```python
from build123d import *

# Parameters (mm, degrees)
SKETCH1_R                 = 26
SKETCH1_R_2               = 17
BOSS_EXTRUDE1_DEPTH       = 6
FILLET1_R                 = 0.2
CUT_EXTRUDE1_START        = 18
SKETCH4_R                 = 2
CUT_EXTRUDE1_DEPTH        = 12
CIRPATTERN1_COUNT         = 6
LPATTERN1_COUNT           = 2
LPATTERN1_PITCH           = 6
LPATTERN1_START           = 18
LPATTERN1_COPY_1_SKETCH_R = 2
LPATTERN1_COPY_1_DEPTH    = 12
LPATTERN1_COPY_2_SKETCH_R = 2
LPATTERN1_COPY_2_DEPTH    = 12
LPATTERN1_COPY_3_SKETCH_R = 2
LPATTERN1_COPY_3_DEPTH    = 12
LPATTERN1_COPY_4_SKETCH_R = 2
LPATTERN1_COPY_4_DEPTH    = 12
LPATTERN1_COPY_5_SKETCH_R = 2
LPATTERN1_COPY_5_DEPTH    = 12


with BuildPart() as part:
    # Sketch1 → Boss-Extrude1 (new, symmetric)
    with BuildSketch(Plane(origin=(0, 0, 0), x_dir=(1, 0, 0), z_dir=(0, 1, 0))):
        with Locations(Location((0, 0, 0), (0, 0, 270))):
            Circle(SKETCH1_R)
        with Locations(Location((0, 0, 0), (0, 0, 270))):
            Circle(SKETCH1_R_2, mode=Mode.SUBTRACT)
    extrude(amount=BOSS_EXTRUDE1_DEPTH, both=True)

    # Sketch3 → Cut-Revolve1 (revolve, cut)
    with BuildSketch(Plane.XY, mode=Mode.PRIVATE) as cut_revolve1_sk:
        Polygon((-26, 0.2), (-26, -0.2), (-25.8, 0), align=None)
    revolve(cut_revolve1_sk.sketch.rotate(Axis((0, -6, 0), (0, 1, 0)), 270), axis=Axis((0, -6, 0), (0, 1, 0)), mode=Mode.SUBTRACT)

    # Fillet1
    fillet1_edges = [part.edges().sort_by_distance(p)[0] for p in [
        (0, -6, -26),
        (0, 6, -26),
    ]]
    fillet(fillet1_edges, radius=FILLET1_R)

    # Sketch4 → Cut-Extrude1 (cut)
    with BuildSketch(Plane.XY.offset(CUT_EXTRUDE1_START)):
        with Locations(Location((0, 3, 0), (0, 0, 180))):
            Circle(SKETCH4_R)
    cut_extrude1 = extrude(amount=CUT_EXTRUDE1_DEPTH, mode=Mode.SUBTRACT)

    # CirPattern1: Cut-Extrude1 ×6 about axis
    cirpattern1_axis = Axis((0, 0, 0), (0, 1, 0))
    for i in range(1, CIRPATTERN1_COUNT):
        add(cut_extrude1.rotate(cirpattern1_axis, i * 360 / CIRPATTERN1_COUNT), mode=Mode.SUBTRACT)

    # LPattern1: Cut-Extrude1 ×2
    with Locations(*[(0, -i * LPATTERN1_PITCH, 0) for i in range(1, LPATTERN1_COUNT)]):
        add(cut_extrude1, mode=Mode.SUBTRACT)

    # LPattern1 copy 1 sketch → LPattern1 copy 1 (cut)
    with BuildSketch(Plane(origin=(0, -6, 0), x_dir=(0.5000000000000001, 0, -0.8660254037844386), z_dir=(0.8660254037844386, 0, 0.5000000000000001)).offset(LPATTERN1_START)):
        with Locations(Location((0, 3, 0), (0, 0, 180))):
            Circle(LPATTERN1_COPY_1_SKETCH_R)
    extrude(amount=LPATTERN1_COPY_1_DEPTH, mode=Mode.SUBTRACT)

    # LPattern1 copy 2 sketch → LPattern1 copy 2 (cut)
    with BuildSketch(Plane(origin=(0, -6, 0), x_dir=(-0.4999999999999998, 0, -0.8660254037844387), z_dir=(0.8660254037844387, 0, -0.4999999999999998)).offset(LPATTERN1_START)):
        with Locations(Location((0, 3, 0), (0, 0, 180))):
            Circle(LPATTERN1_COPY_2_SKETCH_R)
    extrude(amount=LPATTERN1_COPY_2_DEPTH, mode=Mode.SUBTRACT)

    # LPattern1 copy 3 sketch → LPattern1 copy 3 (cut)
    with BuildSketch(Plane(origin=(0, -6, 0), x_dir=(-1, 0, 0), z_dir=(0, 0, -1)).offset(LPATTERN1_START)):
        with Locations(Location((0, 3, 0), (0, 0, 180))):
            Circle(LPATTERN1_COPY_3_SKETCH_R)
    extrude(amount=LPATTERN1_COPY_3_DEPTH, mode=Mode.SUBTRACT)

    # LPattern1 copy 4 sketch → LPattern1 copy 4 (cut)
    with BuildSketch(Plane(origin=(0, -6, 0), x_dir=(-0.5000000000000004, 0, 0.8660254037844384), z_dir=(-0.8660254037844384, 0, -0.5000000000000004)).offset(LPATTERN1_START)):
        with Locations(Location((0, 3, 0), (0, 0, 180))):
            Circle(LPATTERN1_COPY_4_SKETCH_R)
    extrude(amount=LPATTERN1_COPY_4_DEPTH, mode=Mode.SUBTRACT)

    # LPattern1 copy 5 sketch → LPattern1 copy 5 (cut)
    with BuildSketch(Plane(origin=(0, -6, 0), x_dir=(0.5000000000000001, 0, 0.8660254037844386), z_dir=(-0.8660254037844386, 0, 0.5000000000000001)).offset(LPATTERN1_START)):
        with Locations(Location((0, 3, 0), (0, 0, 180))):
            Circle(LPATTERN1_COPY_5_SKETCH_R)
    extrude(amount=LPATTERN1_COPY_5_DEPTH, mode=Mode.SUBTRACT)


solid = part.part
```
Design review of the part built by this model. Coordinates are the model's own, in mm. A direction names the side the tool comes from. Round coordinates to 2 decimals unless told otherwise and drop trailing zeros. Write each loop counter-clockwise with the first axis right and the second up, starting at its lowest first coordinate (ties: lowest second). Pieces come first, ordered by that corner, then holes.
Item 1: For probe 1 along Y at (x, z) = (0, 20); probe 2 along Y at (x, z) = (17.5, 11); probe 3 along X at (y, z) = (-3.25, -8), list the stretches that pass through material, from the lowest coordinate up.
Item 2: We need section D-D on z = 9. State how many separate pieces and enclosed holes the cut face has, and give its area (3 significant figures).
Item 3: We need section C-C on y = -3. Write out the cut boundary in (x, z), and give its area (3 significant figures).
Item 4: For faces 1 (the cylindrical face through (16.855, -0.084, -2.213)), 2 (the flat face through (0, 3, 18)), 3 (the flat face through (15.6, -3.03, 8.98)), 4 (the cylindrical face through (0, -1, -22)), list the 3-axis set-ups (+Z, -Z, +X, -X, +Y, -Y) from which the entire face can be reached by the end or side of a thin tool; tool diameter is ignored.
Item 5: The part is to be moulded in two halves that separate along Z. For faces 5 (the flat face through (0, -3, -18)), 6 (the cylindrical face through (18.08, 3.77, 12.57)), 7 (the cylindrical face through (0, 5, 22)), say which applies: +Z half, -Z half, draft (parallel to the pull), parting line (faces both ways), or undercut.
Item 6: Clearance check with flat-ended pins moving along their axes: pin 1 Ø1.2 at (x, y) = (-0.5, -2.5) entering from -Z; pin 2 Ø2 at (x, y) = (1, 2.5) entering from +Z; pin 3 Ø1 at (y, z) = (3, 0) entering from -X. State where each tip first meets the part, or that it passes through.
Item 7: We need section B-B on z = 0. Write out the cut boundary in (x, y), and give its area (3 significant figures).
Returned:
1. probe 1: y = -6 to -5, -1 to 1, 5 to 6
1. probe 2: y = -6 to -4.84, -1.16 to 1.16, 4.84 to 6
1. probe 3: x = -24.74 to -17.83, -16.17 to -15, 15 to 16.17, 17.83 to 24.74
2. separate pieces: 2
2. enclosed holes: 4
2. area: 189 mm2
3. outline: (-23.45, -11.23) - (-16.59, -7.27) - (-14.59, -10.73) - (-21.45, -14.69) arc R26 ccw to (-2, -25.92) - (-2, -18) - (2, -18) - (2, -25.92) arc R26 ccw to (21.45, -14.69) - (14.59, -10.73) - (16.59, -7.27) - (23.45, -11.23) arc R26 ccw to (23.45, 11.23) - (16.59, 7.27) - (14.59, 10.73) - (21.45, 14.69) arc R26 ccw to (2, 25.92) - (2, 18) - (-2, 18) - (-2, 25.92) arc R26 ccw to (-21.45, 14.69) - (-14.59, 10.73) - (-16.59, 7.27) - (-23.45, 11.23) arc R26 ccw to start; hole circle Ø34 at (0, 0)
3. area: 1,020 mm2
4. face 1: +Y, -Y
4. face 2: +Z
4. face 3: none
4. face 4: -Z
5. face 5: -Z half
5. face 6: undercut
5. face 7: draft
6. pin 1: stops at z = -18
6. pin 2: stops at z = 25.96
6. pin 3: stops at x = -26
7. outline: (-26, -5.8) arc R0.2 ccw to (-25.8, -6) - (-17, -6) - (-17, 6) - (-25.8, 6) arc R0.2 ccw to (-26, 5.8) - (-26, 0.2) - (-25.8, 0) - (-26, -0.2) - close; (17, -6) - (25.8, -6) arc R0.2 ccw to (26, -5.8) - (26, -0.2) - (25.8, 0) - (26, 0.2) - (26, 5.8) arc R0.2 ccw to (25.8, 6) - (17, 6) - close
7. area: 216 mm2
